from build123d import *

# Parameters (mm, degrees)
BOSS_EXTRUDE2_DEPTH = 1
CUT_EXTRUDE2_REACH  = 8.191
SKETCH4_R           = 3


with BuildPart() as part:
    # Sketch2 → Boss-Extrude2 (new body)
    with BuildSketch(Plane(origin=(0, 0, 0), x_dir=(1, 0, 0), z_dir=(0, 1, 0))):
        Polygon((0, 4.618802154), (-4, 2.309401077), (-4, -2.309401077), (0, -4.618802154), (4, -2.309401077), (4, 2.309401077), align=None)
    extrude(amount=BOSS_EXTRUDE2_DEPTH)

    # Sketch4 → Cut-Extrude2 (cut, up to next)
    with BuildSketch(Plane(origin=(0, 1, 0), x_dir=(1, 0, 0), z_dir=(0, 1, 0)), mode=Mode.PRIVATE) as cut_extrude2_sk1:
        with Locations(Location((0, 0, 0), (0, 0, 270))):
            Circle(SKETCH4_R)
    cut_extrude2_tool1 = extrude(cut_extrude2_sk1.sketch, amount=-CUT_EXTRUDE2_REACH, mode=Mode.PRIVATE) & part.part
    add(cut_extrude2_tool1.solids().sort_by_distance((0, 1, 0))[0], mode=Mode.SUBTRACT)


solid = part.part
Geometry check sheet. Reference: the model listing, model coordinates, mm. Give positions to 0.01 mm unless a question says otherwise; leave off trailing zeros. Loops run counter-clockwise (first coordinate to the right, second up) from the corner with the lowest first, then second, coordinate; pieces in that order, holes last. Notation, with made-up numbers: (14, -7) -> (36, -7) arc R26 ccw to (36, 25) -> close; hole circle Ø6 at (9.25, 12.5). An arc over 180 degrees is marked (long way). Answer in a Markdown table with one row per item. Add a question column.
1) Cross-section at A-A on z = 0. Record the boundary of the cut face in (x, y).
2) Cross-section at C-C on x = -2.5. Record the boundary of the cut face in (y, z), and give its area (3 significant figures).
3) Material ranges on probe 1 along X at (y, z) = (0.25, 0); probe 2 along X at (y, z) = (0.7, 2); probe 3 along Z at (x, y) = (-2.5, 0.7), recorded low to high. Write a range as from..to.
4) Cross-section at D-D on z = -3.5. Record the boundary of the cut face in (x, y), and give its area (3 significant figures).
5) Gauge pin test, flat end, axial feed: P1, Ø2, axis at x = 1, z = 1, coming from the -Y side. Record the tip position at first contact, or that the pin passes through.
6) Draft check along X on faces 1 (the face through (2.028, 0.493, -3.448)), 2 (the face through (0.9, 0.51, 2.86)), 3 (the face through (-4, 0.5, 0)), 4 (the face through (1, 0, 3)). Enter one of: pulls with the +X half, pulls with the -X half, needs draft (parallel to the pull), parting line crosses it, or undercut.
7) Cross-section at B-B on y = 0.5. Record the boundary of the cut face in (x, z).
Outcome:
| question | item | result |
|---|---|---|
| 1 | outline | (-4, 0) -> (-3, 0) -> (-3, 1) -> (-4, 1) -> close; (3, 0) -> (4, 0) -> (4, 1) -> (3, 1) -> close |
| 2 | outline | (0, -3.18) -> (1, -3.18) -> (1, -1.66) -> (0, -1.66) -> close; (0, 1.66) -> (1, 1.66) -> (1, 3.18) -> (0, 3.18) -> close |
| 2 | area | 3.03 mm^2 |
| 3 | probe 1 | x = -4..-3, 3..4 |
| 3 | probe 2 | x = -4..-2.24, 2.24..4 |
| 3 | probe 3 | z = -3.18..-1.66, 1.66..3.18 |
| 4 | outline | (-1.94, 0) -> (1.94, 0) -> (1.94, 1) -> (-1.94, 1) -> close |
| 4 | area | 3.88 mm^2 |
| 5 | P1 | passes through |
| 6 | face 1 | pulls with the +X half |
| 6 | face 2 | undercut |
| 6 | face 3 | pulls with the -X half |
| 6 | face 4 | needs draft |
| 7 | outline | (-4, -2.31) -> (0, -4.62) -> (4, -2.31) -> (4, 2.31) -> (0, 4.62) -> (-4, 2.31) -> close; hole circle Ø6 at (0, 0) |
